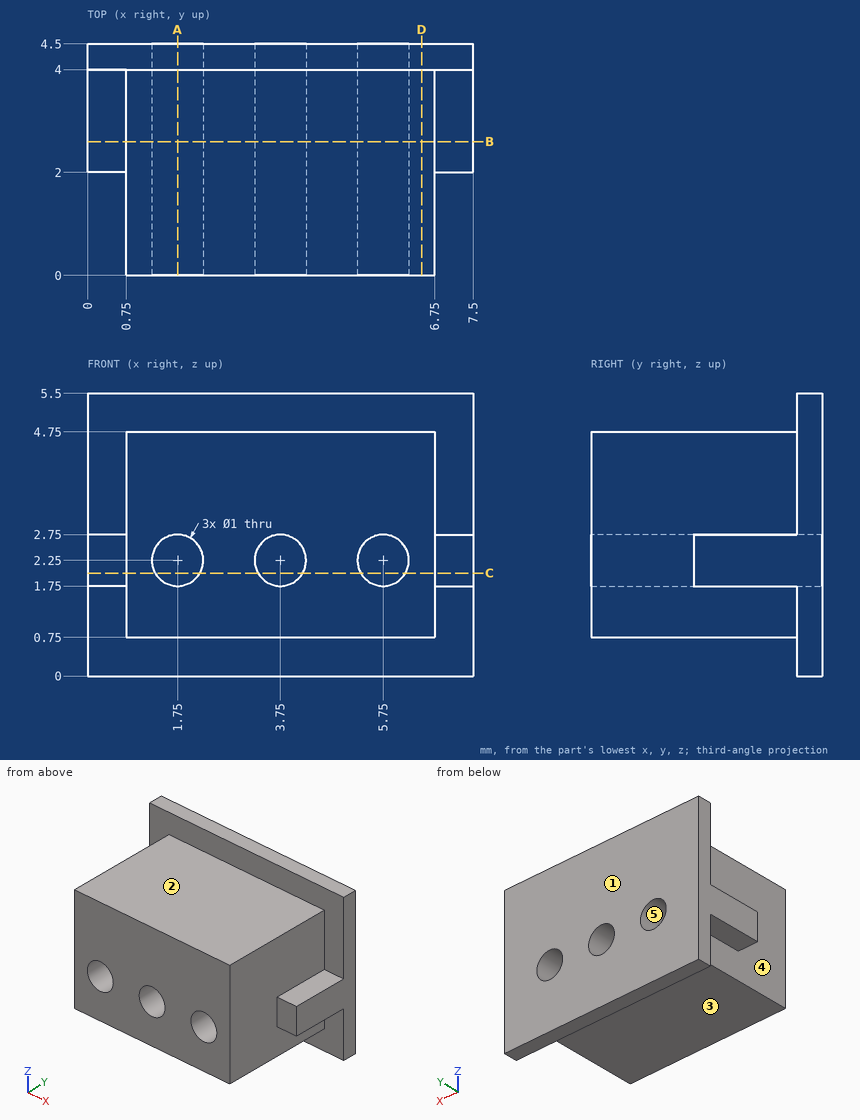
Study the drawing (mm; zero at the part's minimum x, y, z) and answer. A direction names the side the tool comes from. Coordinates: 2 decimals unless noted, no trailing zeros. Write each loop counter-clockwise with the first axis right and the second up, starting at its lowest first coordinate (ties: lowest second). Pieces come first, ordered by that corner, then holes. Notation, with made-up numbers: (76.5, 17.5) - (83.5, 17.5) arc R19 ccw to (83.5, 28.5) - close; hole circle Ø4 at (52, 57.5). An arc over 180 degrees is marked (long way). Answer as a JSON object with one key per item and string values.
Q1. For a pull along Z with two mould halves and no side action, classify the marked faces 3, 4 and 5 as pulls with the +Z half, pulls with the -Z half, needs draft (parallel to the pull), parting line crosses it, or undercut.
Results list:
{"face 3": "pulls with the -Z half", "face 4": "needs draft", "face 5": "undercut"}
Q2. Which of the six approach directions +Z, -Z, +X, -X, +Y, -Y give full straight-line access (tool end or side, diameter ignored) to the marked faces 1 and 2?
Results list:
{"face 1": "+Z, -Z, +X, -X, +Y", "face 2": "+Z, +X, -X, -Y"}
Q3. Given pin 1 Ø2 at (y, z) = (2, 3.5) entering from +X; pin 2 Ø0.6 at (x, y) = (7, 3) entering from +Z, each flat-ended and moving along its own axis, determine where each tip first touches the part or whether it passes through.
Results list:
{"pin 1": "stops at x = 7.5", "pin 2": "stops at z = 4.75"}
Q4. Find section A-A (x = 1.75). Write down the section's boundary in (y, z).
Results list:
{"outline": "(0, 0.75) - (4, 0.75) - (4, 0) - (4.5, 0) - (4.5, 1.75) - (0, 1.75) - close; (0, 2.75) - (4.5, 2.75) - (4.5, 5.5) - (4, 5.5) - (4, 4.75) - (0, 4.75) - close"}
Q5. Find section B-B (y = 2.6). Write down the section's boundary in (x, z).
Results list:
{"outline": "(0, 1.75) - (0.75, 1.75) - (0.75, 0.75) - (6.75, 0.75) - (6.75, 1.75) - (7.5, 1.75) - (7.5, 2.75) - (6.75, 2.75) - (6.75, 4.75) - (0.75, 4.75) - (0.75, 2.75) - (0, 2.75) - close; hole circle Ø1 at (1.75, 2.25); hole circle Ø1 at (3.75, 2.25); hole circle Ø1 at (5.75, 2.25)"}
Q6. Consider L1, parallel to X at y = 3.4, z = 2.25; L2, parallel to X at y = 1.5, z = 2.25; L3, parallel to Z at x = 7.25, y = 3.25. Determine where each line is inside the solid, lowest interval first. Write a range as from..to.
Results list:
{"L1": "x = 0..1.25, 2.25..3.25, 4.25..5.25, 6.25..7.5", "L2": "x = 0.75..1.25, 2.25..3.25, 4.25..5.25, 6.25..6.75", "L3": "z = 1.75..2.75"}
Q7. Find section D-D (x = 6.5). Write down the section's boundary in (y, z).
Results list:
{"outline": "(0, 0.75) - (4, 0.75) - (4, 0) - (4.5, 0) - (4.5, 5.5) - (4, 5.5) - (4, 4.75) - (0, 4.75) - close"}
Q8. Find section C-C (z = 2). Write down the section's boundary in (x, y), plus the area to 3 significant figures.
Results list:
{"outline": "(0, 2) - (0.75, 2) - (0.75, 0) - (1.32, 0) - (1.32, 4.5) - (0, 4.5) - close; (2.18, 0) - (3.32, 0) - (3.32, 4.5) - (2.18, 4.5) - close; (4.18, 0) - (5.32, 0) - (5.32, 4.5) - (4.18, 4.5) - close; (6.18, 0) - (6.75, 0) - (6.75, 2) - (7.5, 2) - (7.5, 4.5) - (6.18, 4.5) - close", "area": "19.1 mm^2"}
